Work out the finished part from the listing and answer in its coordinate system (mm). Round coordinates to 2 decimals unless told otherwise and drop trailing zeros. Write each loop counter-clockwise with the first axis right and the second up, starting at its lowest first coordinate (ties: lowest second). Pieces come first, ordered by that corner, then holes. Notation, with made-up numbers: (50, -7.75) - (69, -7.75) arc R24 ccw to (69, 29.25) - close; hole circle Ø5 at (63, 77.25). An arc over 180 degrees is marked (long way). Answer as a JSON object with one key per item and string values.
```python
from build123d import *

# Parameters (mm, degrees)
BOSS_EXTRUDE1_DEPTH     = 240.2
CUT_EXTRUDE3_DEPTH      = 540.188032545
CUT_EXTRUDE3_DEPTH_BACK = 540.188032545
SKETCH2_OUTSIDE_W       = 932.224
SKETCH2_OUTSIDE_H       = 412.374
SKETCH2_OUTSIDE_W_2     = 760.049325768
SKETCH2_OUTSIDE_H_2     = 72.06
CUT_EXTRUDE4_DEPTH      = 540.188032545
CUT_EXTRUDE5_DEPTH      = 540.182188788
CUT_EXTRUDE5_DEPTH_BACK = 540.182188788
SKETCH4_W               = 3
SKETCH4_H               = 10


with BuildPart() as part:
    # Sketch1 → Boss-Extrude1 (new body)
    with BuildSketch(Plane.XY):
        Polygon((0, 0), (380.024662884, 293.716437401), (376.967027683, 297.672555066), (0, 6.319326703), (-376.967027683, 297.672555066), (-380.024662884, 293.716437401), align=None)
    extrude(amount=-BOSS_EXTRUDE1_DEPTH)

    # Sketch2 outside → Cut-Extrude3 (cut, two sides: drawn at the far end of the back side and taken through both)
    with BuildSketch(Plane(origin=(0, 0, 0), x_dir=(1, 0, 0), z_dir=(0, 1, 0)).offset(-CUT_EXTRUDE3_DEPTH_BACK)):
        with Locations((0, 120.1)):
            Rectangle(SKETCH2_OUTSIDE_W, SKETCH2_OUTSIDE_H)
        with Locations((0, 204.17)):
            Rectangle(SKETCH2_OUTSIDE_W_2, SKETCH2_OUTSIDE_H_2, mode=Mode.SUBTRACT)
    extrude(amount=CUT_EXTRUDE3_DEPTH + CUT_EXTRUDE3_DEPTH_BACK, mode=Mode.SUBTRACT)

    # Sketch3 → Cut-Extrude4 (cut, through all)
    with BuildSketch(Plane(origin=(0, 0, 0), x_dir=(1, 0, 0), z_dir=(0, 1, 0))):
        Polygon((41.603860398, 240.2), (0, 168.14), (380.024662884, 168.14), (380.024662884, 240.2), align=None)
        Polygon((41.603860398, 240.2), (-41.603860398, 240.2), (0, 168.14), align=None)
    extrude(amount=CUT_EXTRUDE4_DEPTH, mode=Mode.SUBTRACT)

    # Sketch4 → Cut-Extrude5 (cut, two sides: drawn at the far end of the back side and taken through both)
    with BuildSketch(Plane(origin=(3.057635201, 3.956117665, 0), x_dir=(0.7912235329674936, -0.6115270401858268, 0), z_dir=(0.6115270401858268, 0.7912235329674936, 0)).offset(-CUT_EXTRUDE5_DEPTH_BACK)):
        with Locations((-250.282219577, 204.17)):
            Rectangle(SKETCH4_W, SKETCH4_H)
    extrude(amount=CUT_EXTRUDE5_DEPTH + CUT_EXTRUDE5_DEPTH_BACK, mode=Mode.SUBTRACT)


solid = part.part
```
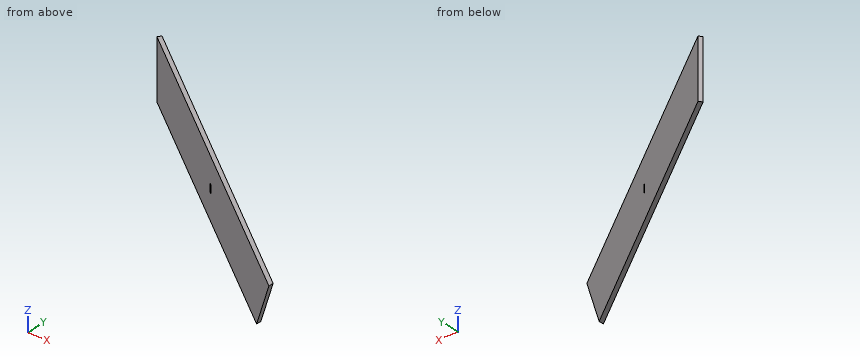
Item 1: Each of these flat-tipped pins is pushed along its axis until it touches: P1, Ø10, axis at x = -333, z = -198.5, coming from the -Y side; P2, Ø12, axis at y = 91.5, z = -194, coming from the -X side; P3, Ø8, axis at y = 153, z = -227.5, coming from the +X side. Where does it stop, or does it pass through?
Results found:
{"P1": "y = 253.51", "P2": "x = -126.15", "P3": "x = -184.61"}
Item 2: A cutting plane is placed at B-B (z = -227.5). Write down the section's boundary in (x, y), and give its area (3 significant figures).
Results found:
{"outline": "(-380.02, 293.72) - (-34.27, 26.49) - (-34.27, 32.81) - (-376.97, 297.67) - close", "area": "2,180 mm²"}
Item 3: A cutting plane is placed at A-A (y = 19). Write down the section's boundary in (x, z), and give its area (3 significant figures).
Results found:
{"outline": "(-24.58, -210.72) - (-16.41, -196.56) - (-16.41, -168.14) - (-24.58, -168.14) - close", "area": "290 mm²"}
Item 4: Consider line 1 along Y through (x, z) = (-41.5, -196.5); line 2 along X through (y, z) = (59.5, -229.5); line 3 along X through (y, z) = (46, -227). Determine where each line is inside the solid, lowest interval first.
Results found:
{"line 1": "32.07 to 38.39", "line 2": "-76.98 to -68.81", "line 3": "-59.52 to -51.34"}
